Design review of the part built by this model. Coordinates are the model's own, in mm. A direction names the side the tool comes from. Give positions to 0.01 mm unless a question says otherwise; leave off trailing zeros. Write each loop counter-clockwise with the first axis right and the second up, starting at its lowest first coordinate (ties: lowest second). Pieces come first, ordered by that corner, then holes. Notation, with made-up numbers: (-6, 49) -> (39, 49) arc R22 ccw to (39, 68) -> close; hole circle Ø10 at (73.25, -33). An arc over 180 degrees is marked (long way). Answer as a JSON object with one key per item and string values.
```python
from build123d import *

# Parameters (mm, degrees)
SKETCH_2_R                         = 35
EXTRUDE_1_DEPTH                    = 3
SKETCH_1_W                         = 3
SKETCH_1_H                         = 8
CUT_EXTRUDE_1_DEPTH                = 3
PATTERN_CIRCULAR_1_COUNT           = 3
PATTERN_CIRCULAR_1_COPY_1_SKETCH_W = 3
PATTERN_CIRCULAR_1_COPY_1_SKETCH_H = 8
PATTERN_CIRCULAR_1_COPY_1_DEPTH    = 3
PATTERN_CIRCULAR_1_COPY_2_SKETCH_W = 3
PATTERN_CIRCULAR_1_COPY_2_SKETCH_H = 8
PATTERN_CIRCULAR_1_COPY_2_DEPTH    = 3
SKETCH_3_R                         = 1.5
CUT_EXTRUDE_3_DEPTH                = 10


with BuildPart() as part:
    # Эскиз2 → Бобышка-Вытянуть1 (new body)
    with BuildSketch(Plane.XY):
        Polygon((0, 51.961524227), (-45, 25.980762114), (-45, -25.980762114), (0, -51.961524227), (45, -25.980762114), (45, 25.980762114), align=None)
        Circle(SKETCH_2_R, mode=Mode.SUBTRACT)
    extrude(amount=EXTRUDE_1_DEPTH)

    # Эскиз1 → Вырез-Вытянуть1 (cut)
    with BuildSketch(Plane.XY):
        with Locations((-38.34595, -17.19729)):
            Rectangle(SKETCH_1_W, SKETCH_1_H)
        with Locations((-38.34595, -9.19729)):
            Rectangle(SKETCH_1_W, SKETCH_1_H)
    cut_extrude_1 = extrude(amount=CUT_EXTRUDE_1_DEPTH, mode=Mode.SUBTRACT)

    # Зеркальное отражение1: Вырез-Вытянуть1 across plane
    add(cut_extrude_1.mirror(Plane.ZX), mode=Mode.SUBTRACT)

    # Круговой массив1: Вырез-Вытянуть1 ×3 about axis
    pattern_circular_1_axis = Axis((0, 0, 0), (0, 0, 1))
    for i in range(1, PATTERN_CIRCULAR_1_COUNT):
        add(cut_extrude_1.rotate(pattern_circular_1_axis, i * 360 / PATTERN_CIRCULAR_1_COUNT), mode=Mode.SUBTRACT)

    # Круговой массив1 copy 1 sketch → Круговой массив1 copy 1 (cut)
    with BuildSketch(Plane(origin=(0, 0, 0), x_dir=(-0.5, 0.866025404, 0), z_dir=(0, 0, 1))):
        with Locations((-38.34595, 17.19729)):
            Rectangle(PATTERN_CIRCULAR_1_COPY_1_SKETCH_W, PATTERN_CIRCULAR_1_COPY_1_SKETCH_H)
        with Locations((-38.34595, 9.19729)):
            Rectangle(PATTERN_CIRCULAR_1_COPY_1_SKETCH_W, PATTERN_CIRCULAR_1_COPY_1_SKETCH_H)
    extrude(amount=PATTERN_CIRCULAR_1_COPY_1_DEPTH, mode=Mode.SUBTRACT)

    # Круговой массив1 copy 2 sketch → Круговой массив1 copy 2 (cut)
    with BuildSketch(Plane(origin=(0, 0, 0), x_dir=(-0.5, -0.866025404, 0), z_dir=(0, 0, 1))):
        with Locations((-38.34595, 17.19729)):
            Rectangle(PATTERN_CIRCULAR_1_COPY_2_SKETCH_W, PATTERN_CIRCULAR_1_COPY_2_SKETCH_H)
        with Locations((-38.34595, 9.19729)):
            Rectangle(PATTERN_CIRCULAR_1_COPY_2_SKETCH_W, PATTERN_CIRCULAR_1_COPY_2_SKETCH_H)
    extrude(amount=PATTERN_CIRCULAR_1_COPY_2_DEPTH, mode=Mode.SUBTRACT)

    # Эскиз3 → Вырез-Вытянуть3 (cut)
    with BuildSketch(Plane.XY):
        with Locations((40, 0)):
            Circle(SKETCH_3_R)
        with Locations((-20, -34.641016151)):
            Circle(SKETCH_3_R)
        with Locations((-20, 34.641016151)):
            Circle(SKETCH_3_R)
    extrude(amount=CUT_EXTRUDE_3_DEPTH, mode=Mode.SUBTRACT)


solid = part.part
```
(1) We need section C-C, the plane x = 8. State the section outline as (y, z) points, then the cut area to 3 significant figures.
Here are the results:
{"outline": "(-47.34, 0) -> (-41.39, 0) -> (-41.39, 3) -> (-47.34, 3) -> close; (-37.93, 0) -> (-34.07, 0) -> (-34.07, 3) -> (-37.93, 3) -> close; (34.07, 0) -> (37.93, 0) -> (37.93, 3) -> (34.07, 3) -> close; (41.39, 0) -> (47.34, 0) -> (47.34, 3) -> (41.39, 3) -> close", "area": "58.8 mm²"}
(2) The part is to be moulded in two halves that separate along Y. For faces 3 (the flat face through (8.4, -41.16, 1.48)), 4 (the flat face through (22.185, -39.153, 1.479)), 5 (the flat face through (45, 0, 1)), say which applies: +Y half, -Y half, draft (parallel to the pull), parting line (faces both ways), or undercut.
Here are the results:
{"face 3": "undercut", "face 4": "-Y half", "face 5": "draft"}
(3) We need section B-B, the plane x = -23.5. State the section outline as (y, z) points, then the cut area to 3 significant figures.
Here are the results:
{"outline": "(-38.39, 0) -> (-25.94, 0) -> (-25.94, 3) -> (-38.39, 3) -> close; (25.94, 0) -> (38.39, 0) -> (38.39, 3) -> (25.94, 3) -> close", "area": "74.7 mm²"}
(4) For faces 1 (the flat face through (31.449, 27.853, 1.479)), 2 (the flat face through (-4, 35, 3)), list the 3-axis set-ups (+Z, -Z, +X, -X, +Y, -Y) from which the entire face can be reached by the end or side of a thin tool; tool diameter is ignored.
Here are the results:
{"face 1": "+Z, -Z", "face 2": "+Z, +X, -X, +Y, -Y"}
(5) We need section D-D, the plane y = -40. State the section outline as (x, z) points.
Here are the results:
{"outline": "(-20.72, 0) -> (4.41, 0) -> (4.41, 3) -> (-20.72, 3) -> close; (10.41, 0) -> (20.72, 0) -> (20.72, 3) -> (10.41, 3) -> close"}
(6) Clearance check with flat-ended pins moving along their axes: pin 1 (1 mm diameter, centred on x = 29, z = 1, fed in from -Y); pin 2 (1.5 mm diameter, centred on x = -8.5, z = 2.5, fed in from -Y); pin 3 (1.5 mm diameter, centred on x = -39, z = 1, fed in from +Y). State where each tip first meets the part, or that it passes through.
Here are the results:
{"pin 1": "stops at y = -35.51", "pin 2": "stops at y = -47.49", "pin 3": "stops at y = 29.88"}
(7) For line 1 along X through (y, z) = (28.5, 1.75); line 2 along Y through (x, z) = (8.5, 0.2); line 3 along Y through (x, z) = (10, 0.4), list the stretches that pass through material, from the lowest coordinate up.
Here are the results:
{"line 1": "x = -40.64 to -20.32, 20.32 to 24.33, 30.33 to 40.64", "line 2": "y = -47.05 to -41.1, -37.64 to -33.95, 33.95 to 37.64, 41.1 to 47.05", "line 3": "y = -46.19 to -40.24, -36.77 to -33.54, 33.54 to 36.77, 40.24 to 46.19"}
(8) We need section A-A, the plane y = 0. State the section outline as (x, z) points, then the cut area to 3 significant figures.
Here are the results:
{"outline": "(-45, 0) -> (-35, 0) -> (-35, 3) -> (-45, 3) -> close; (35, 0) -> (38.5, 0) -> (38.5, 3) -> (35, 3) -> close; (41.5, 0) -> (45, 0) -> (45, 3) -> (41.5, 3) -> close", "area": "51.0 mm²"}
